Work out the finished part from the listing and answer in its coordinate system (mm). Coordinates: 2 decimals unless noted, no trailing zeros. Order: outer loops, then holes, each group sorted by start corner. A loop starts at its lowest first (then second) coordinate and runs counter-clockwise, first axis right, second up. Notation, with made-up numbers: M 21.5,73.5 L 30.5,73.5 A17 cw 30.5,88.5 Z; hole C -14.75,44.25 d6. An arc over 180 degrees is marked long. Write item = value, one per line. Start each with the question number.
Q1. Find section A-A on y = 0.9. Give the number of separate pieces and of enclosed holes in the cut face, and give its area (3 significant figures).
Q2. Straight lines are drawn through the part: line 1 along Z through (x, y) = (115, 1.05); line 2 along X through (y, z) = (0.35, -30.5). For each, find the intervals that lie inside material, in ascending order.
Q3. Find section B-B on x = 9.5. Give the vertices of the cut face in (y, z) (3 decimals).
Q4. Each of these flat-tipped pins is pushed along its axis until it touches: P1, Ø1.6, axis at y = 1.5, z = -2, coming from the +X side; P2, Ø1.6, axis at x = 3, y = 2.5, coming from the +Z side. Where does it stop, or does it pass through?
```python
from build123d import *

# Parameters (mm, degrees)
SKETCH2_W          = 250
SKETCH2_H          = 250
BASE_DEPTH         = 3.175
SKETCH3_W          = 8.6
SKETCH3_H          = 15.35
HOLES_DEPTH        = 10
SKETCH4_W          = 45.1
SKETCH4_H          = 25.1
SKETCH4_W_2        = 20.378913316
SKETCH4_H_2        = 45.1
SKETCH4_H_3        = 20.378913316
JIGSAW_DEPTH       = 10
STANDOFF_HOLES_D   = 2.5
STANDOFF_HOLES_2_D = 2.5


with BuildPart() as part:
    # Sketch2 → Base (new body)
    with BuildSketch(Plane(origin=(0, 0, 0), x_dir=(1, 0, 0), z_dir=(0, 1, 0))):
        Rectangle(SKETCH2_W, SKETCH2_H)
    extrude(amount=BASE_DEPTH)

    # Sketch3 → Holes (cut)
    with BuildSketch(Plane(origin=(0, 3.175, 0), x_dir=(1, 0, 0), z_dir=(0, 1, 0))):
        with Locations((-43.75, 35.675)):
            Rectangle(SKETCH3_W, SKETCH3_H)
        with Locations((-43.75, -35.675)):
            Rectangle(SKETCH3_W, SKETCH3_H)
        with Locations((43.75, -35.675)):
            Rectangle(SKETCH3_W, SKETCH3_H)
        with Locations((43.75, 35.675)):
            Rectangle(SKETCH3_W, SKETCH3_H)
    extrude(amount=-HOLES_DEPTH, mode=Mode.SUBTRACT)

    # Sketch4 → Jigsaw (cut)
    with BuildSketch(Plane(origin=(0, 3.175, 0), x_dir=(1, 0, 0), z_dir=(0, 1, 0))):
        with Locations((0, 125)):
            Rectangle(SKETCH4_W, SKETCH4_H)
        with Locations((-125, 0)):
            Rectangle(SKETCH4_W_2, SKETCH4_H_2)
        with Locations((125, 0)):
            Rectangle(SKETCH4_W_2, SKETCH4_H_2)
        with Locations((0, -125)):
            Rectangle(SKETCH4_W, SKETCH4_H_3)
    extrude(amount=-JIGSAW_DEPTH, mode=Mode.SUBTRACT)

    # Standoff Holes (through all)
    with Locations(Plane(origin=(0, 3.175, 0), x_dir=(1, 0, 0), z_dir=(0, 1, 0))):
        with Locations((-115, 115)):
            Hole(STANDOFF_HOLES_D / 2)

    # Standoff Holes 2 (through all)
    with Locations(Plane(origin=(0, 3.175, 0), x_dir=(1, 0, 0), z_dir=(0, 1, 0))):
        with Locations((115, 115), (115, -115), (-115, -115)):
            Hole(STANDOFF_HOLES_2_D / 2)


solid = part.part
```
Findings below:
q1.separate_pieces = 1
q1.enclosed_holes = 8
q1.area = 60,000 mm^2
q2.line_1 = -125 to -116.25, -113.75 to -22.55, 22.55 to 113.75, 116.25 to 125
q2.line_2 = -125 to -48.05, -39.45 to 39.45, 48.05 to 125
q3.outline = M 0,-112.45 L 3.175,-112.45 L 3.175,114.811 L 0,114.811 Z
q4.P1 = 114.81
q4.P2 = 114.81
